Can you work these out from the drawing? Everything is in mm from the part's minimum corner. Round coordinates to 2 decimals unless told otherwise and drop trailing zeros. Write each loop counter-clockwise with the first axis right and the second up, starting at its lowest first coordinate (ties: lowest second). Pieces come first, ordered by that corner, then holes. Notation, with made-up numbers: (-36.75, -22.5) -> (4.25, -22.5) arc R33 ccw to (4.25, 16.5) -> close; hole circle Ø8 at (63, 35.5). An arc over 180 degrees is marked (long way). One line per question, with ' | ' between items. Start each with the question number.
1. Thinking about a two-plate mould opening in X: for the marked faces 1, 2 and 3, which applies, released by +X, released by -X, zero draft, split by the parting line, or undercut?
2. Imagine slicing it at A-A, the plane x = 8.89. List the corners of the cut face in (y, z) for me.
3. Imagine slicing it at D-D, the plane z = 8. List the corners of the cut face in (x, y) for me, and give its area (3 significant figures).
4. Imagine slicing it at C-C, the plane y = 3.25. State how many separate pieces and enclosed holes the cut face has, and give its area (3 significant figures).
5. For pin 1 Ø1.4 at (x, z) = (21.59, 15.24) entering from +Y, with a flat end and sliding along its axis, tell me the tip position at first contact or that it passes through.
6. If I drill on line 1 along Z through (x, y) = (8.89, 2.5); line 2 along X through (y, z) = (5.5, 14.5) (1 decimal); line 3 along X through (y, z) = (4.75, 3.5) (1 decimal), over which ranges is the centre line in solid material (lowest first)? Write a range as [from, to].
7. Imagine slicing it at B-B, the plane z = 15.24. List the corners of the cut face in (x, y) for me.
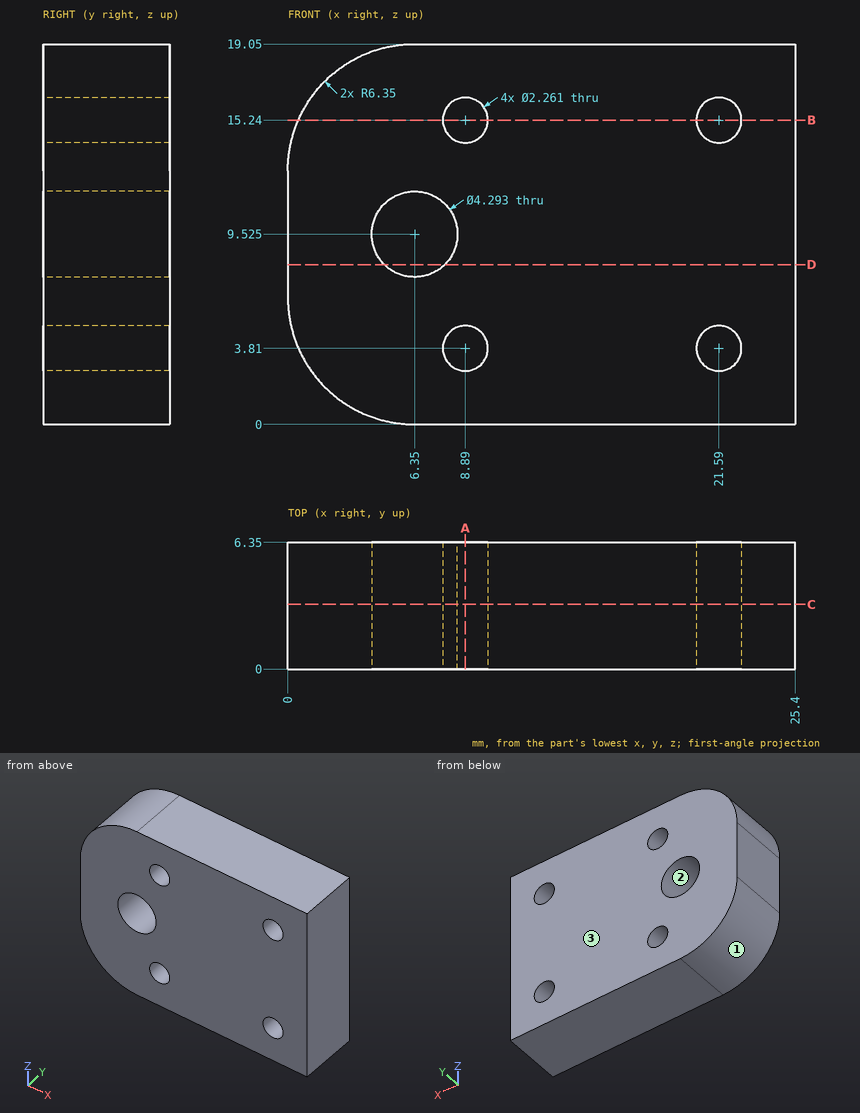
Geometry results:
1) face 1: released by -X | face 2: undercut | face 3: zero draft
2) outline: (0, 0) -> (6.35, 0) -> (6.35, 2.68) -> (0, 2.68) -> close; (0, 4.94) -> (6.35, 4.94) -> (6.35, 14.11) -> (0, 14.11) -> close; (0, 16.37) -> (6.35, 16.37) -> (6.35, 19.05) -> (0, 19.05) -> close
3) outline: (0, 0) -> (4.84, 0) -> (4.84, 6.35) -> (0, 6.35) -> close; (7.86, 0) -> (25.4, 0) -> (25.4, 6.35) -> (7.86, 6.35) -> close | area: 142 mm2
4) separate pieces: 1 | enclosed holes: 5 | area: 436 mm2
5) pin 1: passes through
6) line 1: z = [0, 2.68], [4.94, 14.11], [16.37, 19.05] | line 2: x = [0.3, 8], [9.7, 20.7], [22.4, 25.4] | line 3: x = [0.7, 7.8], [10, 20.5], [22.7, 25.4]
7) outline: (0.53, 0) -> (7.76, 0) -> (7.76, 6.35) -> (0.53, 6.35) -> close; (10.02, 0) -> (20.46, 0) -> (20.46, 6.35) -> (10.02, 6.35) -> close; (22.72, 0) -> (25.4, 0) -> (25.4, 6.35) -> (22.72, 6.35) -> close
